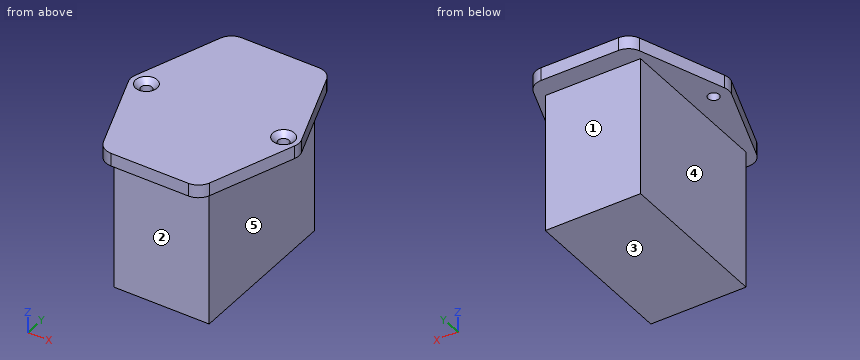
```python
from build123d import *

# Parameters (mm, degrees)
SKETCH1_W                                       = 27.75
SKETCH1_H                                       = 46.5
BOSS_EXTRUDE1_DEPTH                             = 40.5
SKETCH2_R                                       = 1.6
BOSS_EXTRUDE2_DEPTH                             = 3.8
CSK_FOR_M3_FLAT_HEAD_MACHINE_SCREW1_D           = 3.2
CSK_FOR_M3_FLAT_HEAD_MACHINE_SCREW1_CSINK_D     = 6.3
CSK_FOR_M3_FLAT_HEAD_MACHINE_SCREW1_CSINK_ANGLE = 90


with BuildPart() as part:
    # Sketch1 → Boss-Extrude1 (new body)
    with BuildSketch(Plane.XY):
        with Locations((13.875, 23.25)):
            Rectangle(SKETCH1_W, SKETCH1_H)
    extrude(amount=BOSS_EXTRUDE1_DEPTH)

    # Sketch2 → Boss-Extrude2 (add)
    with BuildSketch(Plane.XY.offset(40.5)):
        with BuildLine():
            Line((2.625, -5.2), (25.125, -5.2))
            ThreePointArc((25.125, -5.2), (27.711215896, -4.382592475), (29.357879644, -2.227327706))
            Line((29.357879644, -2.227327706), (38.107879644, 22.022672294))
            ThreePointArc((38.107879644, 22.022672294), (38.375, 23.55), (38.107879644, 25.077327706))
            Line((38.107879644, 25.077327706), (29.357879644, 49.327327706))
            ThreePointArc((29.357879644, 49.327327706), (27.711215896, 51.482592475), (25.125, 52.3))
            Line((25.125, 52.3), (2.625, 52.3))
            ThreePointArc((2.625, 52.3), (0.038784104, 51.482592475), (-1.607879644, 49.327327706))
            Line((-1.607879644, 49.327327706), (-10.357879644, 25.077327706))
            ThreePointArc((-10.357879644, 25.077327706), (-10.625, 23.55), (-10.357879644, 22.022672294))
            Line((-10.357879644, 22.022672294), (-1.607879644, -2.227327706))
            ThreePointArc((-1.607879644, -2.227327706), (0.038784104, -4.382592475), (2.625, -5.2))
        make_face()
        with Locations((-6.125, 23.55)):
            Circle(SKETCH2_R, mode=Mode.SUBTRACT)
        with Locations((33.875, 23.55)):
            Circle(SKETCH2_R, mode=Mode.SUBTRACT)
    extrude(amount=BOSS_EXTRUDE2_DEPTH)

    # CSK for M3 Flat Head Machine Screw1 (through all)
    with Locations(Plane.XY.offset(44.3)):
        with Locations((-6.125, 23.55), (33.875, 23.55)):
            CounterSinkHole(CSK_FOR_M3_FLAT_HEAD_MACHINE_SCREW1_D / 2, CSK_FOR_M3_FLAT_HEAD_MACHINE_SCREW1_CSINK_D / 2, counter_sink_angle=CSK_FOR_M3_FLAT_HEAD_MACHINE_SCREW1_CSINK_ANGLE)


solid = part.part
```
The model under review builds one solid part; all positions refer to its coordinate system, in mm. Face numbers are marked on the shaded views. A direction names the side the tool comes from. Round coordinates to 2 decimals unless told otherwise and drop trailing zeros. Loops run counter-clockwise (first coordinate to the right, second up) from the corner with the lowest first, then second, coordinate; pieces in that order, holes last. Notation, with made-up numbers: M 79.5,19 L 116.5,19 A18 ccw 116.5,48 Z; hole C 29.5,47.5 d1. An arc over 180 degrees is marked long. Answer as a JSON object with one key per item and string values.
(1) Clearance check with flat-ended pins moving along their axes: P1, Ø2, axis at y = 40, z = 12.5, coming from the +X side; P2, Ø1.5, axis at y = 18.5, z = 32.5, coming from the -X side; P3, Ø8.5, axis at x = 9, z = 13, coming from the +Y side. State where each tip first meets the part, or that it passes through.
Resolved:
{"P1": "x = 27.75", "P2": "x = 0", "P3": "y = 46.5"}
(2) To check wall thickness, follow line 1 along X through (y, z) = (23.55, 42) (3 decimals); line 2 along X through (y, z) = (23, 42); line 3 along Y through (x, z) = (10, 14). State the ranges of each line that lie inside material, in increasing order.
Resolved:
{"line 1": "-10.625 to -7.725, -4.525 to 32.275, 35.475 to 38.375", "line 2": "-10.59 to -7.63, -4.62 to 32.37, 35.38 to 38.34", "line 3": "0 to 46.5"}
(3) Take a section at C-C on z = 41.5. Give the boundary of the cut face in (x, y) (3 decimals), and give its area (3 significant figures).
Resolved:
{"outline": "M -10.358,22.023 L -1.608,-2.227 A4.5 ccw 2.625,-5.2 L 25.125,-5.2 A4.5 ccw 29.358,-2.227 L 38.108,22.023 A4.5 ccw 38.108,25.077 L 29.358,49.327 A4.5 ccw 25.125,52.3 L 2.625,52.3 A4.5 ccw -1.608,49.327 L -10.358,25.077 A4.5 ccw Z; hole C -6.125,23.55 d3.2; hole C 33.875,23.55 d3.2", "area": "2,230 mm²"}
(4) Tool access review of the marked faces 1, 2, 3, 4 and 5: name each direction out of +Z, -Z, +X, -X, +Y, -Y from which nothing blocks a thin tool from reaching the whole face with its end or side.
Resolved:
{"face 1": "-Z, +X, -X, +Y", "face 2": "-Z, +X, -X, -Y", "face 3": "-Z, +X, -X, +Y, -Y", "face 4": "-Z, -X, +Y, -Y", "face 5": "-Z, +X, +Y, -Y"}
(5) Take a section at B-B on x = 14.5. Give the boundary of the cut face in (y, z).
Resolved:
{"outline": "M -5.2,40.5 L 0,40.5 L 0,0 L 46.5,0 L 46.5,40.5 L 52.3,40.5 L 52.3,44.3 L -5.2,44.3 Z"}
(6) Take a section at A-A on y = 23.55. Give the boundary of the cut face in (x, z) (3 decimals), and give its area (3 significant figures).
Resolved:
{"outline": "M -10.625,40.5 L -7.725,40.5 L -7.725,42.75 L -9.275,44.3 L -10.625,44.3 Z; M -4.525,40.5 L 0,40.5 L 0,0 L 27.75,0 L 27.75,40.5 L 32.275,40.5 L 32.275,42.75 L 30.725,44.3 L -2.975,44.3 L -4.525,42.75 Z; M 35.475,40.5 L 38.375,40.5 L 38.375,44.3 L 37.025,44.3 L 35.475,42.75 Z", "area": "1,280 mm²"}
(7) Take a section at D-D on y = 10.5. Give the boundary of the cut face in (x, z).
Resolved:
{"outline": "M -6.2,40.5 L 0,40.5 L 0,0 L 27.75,0 L 27.75,40.5 L 33.95,40.5 L 33.95,44.3 L -6.2,44.3 Z"}
